Model file for the job. Use its own axes, mm. Coordinates: 2 decimals unless noted, no trailing zeros. Write each loop counter-clockwise with the first axis right and the second up, starting at its lowest first coordinate (ties: lowest second). Pieces come first, ordered by that corner, then holes.
Q1. Drill centre lines: probe 1 along X at (y, z) = (-12, 11); probe 2 along X at (y, z) = (22, 22.5). Where is each one in solid material? Low to high.
Q2. Band-saw the part on B-B, the plane x = -17. Write the cut outline in (y, z).
Q3. Band-saw the part on C-C, the plane y = -14. Write the cut outline in (x, z), plus the area to 3 significant figures.
Q4. Pin check, flat tips, straight feed: P1, Ø1.5, axis at y = -18.5, z = 15, coming from the +X side; P2, Ø3, axis at y = 13.5, z = 44.5, coming from the -X side. Stop position of each tip, or through.
from build123d import *

# Parameters (mm, degrees)
F1_DEPTH = 52
F2_R     = 5
F3_R     = 4.99999


# Not quite as in the source:
# - a fillet or chamfer is up to 0.001 mm smaller than in the source, because OpenCascade refuses the exact size


with BuildPart() as f1:
    # F0 (on Top) → F1 (new body)
    with BuildSketch(Plane.XY):
        Polygon((15, 25), (-15, 25), (-15, 15), (-25, 15), (-25, -15), (-15, -15), (-15, -25), (15, -25), (15, -15), (25, -15), (25, 15), (15, 15), align=None)
    extrude(amount=F1_DEPTH)

    # F2
    f2_edges = [f1.edges().sort_by_distance(p)[0] for p in [
        (-15, -15, 26),
        (15, -15, 26),
        (15, 15, 26),
        (-15, 15, 26),
    ]]
    fillet(f2_edges, radius=F2_R)

    # F3 (radius 5 in the source; OpenCascade refuses exactly that, so slightly less here)
    f3_edges = [f1.edges().sort_by_distance(p)[0] for p in [
        (25, 15, 26),
        (-15, 25, 26),
        (-25, 15, 26),
        (25, -15, 26),
        (15, -25, 26),
        (-15, -25, 26),
        (-25, -15, 26),
        (15, 25, 26),
    ]]
    fillet(f3_edges, radius=F3_R)


solid = f1.part
Answer sheet:
1. probe 1: x = -24.58 to 24.58
1. probe 2: x = -14.58 to 14.58
2. outline: (-16, 0) - (16, 0) - (16, 52) - (-16, 52) - close
3. outline: (-23, 0) - (23, 0) - (23, 52) - (-23, 52) - close
3. area: 2,390 mm2
4. P1: stops at x = 15.53
4. P2: stops at x = -24.58
